from build123d import *

# Parameters (mm, degrees)
SKETCH8_R               = 35
BOSS_EXTRUDE3_DEPTH     = 1
BOSS_EXTRUDE4_START     = -53.594889
SKETCH9_R               = 5
BOSS_EXTRUDE4_DEPTH     = 113.594889
CUT_EXTRUDE2_START      = -20.791267
SKETCH10_R              = 4
CUT_EXTRUDE2_DEPTH      = 20.791267
SKETCH11_R              = 1.5
CUT_EXTRUDE3_DEPTH      = 73.971936727
BOSS_EXTRUDE5_REACH     = 74.567
SKETCH13_W              = 88.883012554
SKETCH13_H              = 5.53578549
CUT_EXTRUDE4_DEPTH      = 110.338922716
SKETCH14_R              = 1
CUT_EXTRUDE5_DEPTH      = 71.019198384
SKETCH15_W              = 75.166178786
SKETCH15_H              = 0.46421451
SKETCH15_W_2            = 75.463979311
CUT_EXTRUDE6_DEPTH      = 109.72955086
CUT_EXTRUDE7_DEPTH      = 109.707210391
CUT_EXTRUDE7_DEPTH_BACK = 109.707210391
SKETCH16_W              = 74.883691919
SKETCH16_H              = 0.2
SKETCH17_W              = 45
SKETCH17_H              = 9.670623623
CUT_EXTRUDE8_DEPTH      = 25
SKETCH18_W              = 45.166247069
SKETCH18_H              = 9.6
BOSS_EXTRUDE6_DEPTH     = 7
SKETCH19_R              = 2
CUT_EXTRUDE9_DEPTH      = 8.2
SKETCH20_W              = 85
SKETCH20_H              = 13.048799846
SKETCH20_W_2            = 85.000162577
SKETCH20_H_2            = 13.925318183
CUT_EXTRUDE10_DEPTH     = 9.6
CUT_EXTRUDE11_DEPTH     = 59.913683698
SKETCH22_R              = 5
SKETCH22_R_2            = 4.8
CUT_EXTRUDE12_DEPTH     = 10.594889107


with BuildPart() as part:
    # Sketch1 → Revolve1 (revolve)
    with BuildSketch(Plane.XY):
        with BuildLine():
            Line((-32.912878475, 10), (-22.912878475, 10))
            ThreePointArc((-22.912878475, 10), (-25, 0), (-22.912878475, -10))
            Line((-22.912878475, -10), (-32.912878475, -10))
            ThreePointArc((-32.912878475, -10), (-34.398511152, 0), (-32.912878475, 10))
        make_face()
    revolve(axis=Axis((0, 0, 0), (0, 1, 0)))

    # Sketch8 → Boss-Extrude3 (add)
    with BuildSketch(Plane.XZ.offset(10)):
        with Locations(Location((0, 0, 0), (0, 0, 270))):
            Circle(SKETCH8_R)
    extrude(amount=BOSS_EXTRUDE3_DEPTH)

    # Sketch9 → Boss-Extrude4 (add)
    with BuildSketch(Plane(origin=(0, 0, 0), x_dir=(0, 0, -1), z_dir=(1, 0, 0)).offset(BOSS_EXTRUDE4_START)):
        Circle(SKETCH9_R)
    extrude(amount=BOSS_EXTRUDE4_DEPTH)

    # Sketch10 → Cut-Extrude2 (cut)
    with BuildSketch(Plane(origin=(60, 0, 0), x_dir=(0, 0, -1), z_dir=(1, 0, 0)).offset(CUT_EXTRUDE2_START)):
        Circle(SKETCH10_R)
    extrude(amount=CUT_EXTRUDE2_DEPTH, mode=Mode.SUBTRACT)

    # Sketch11 → Cut-Extrude3 (cut, through all)
    with BuildSketch(Plane(origin=(0, 0.188776478, -4.996435073), x_dir=(-1, 0, 0), z_dir=(0, 0.03775529554410709, -0.9992870146551377))):
        with Locations(Location((-55, 0, 0), (0, 0, 90))):
            Circle(SKETCH11_R)
    extrude(amount=-CUT_EXTRUDE3_DEPTH, mode=Mode.SUBTRACT)

    # Boss-Extrude5: up to this face of the body (flat: up to its plane)
    boss_extrude5_end = Plane(part.part.faces().sort_by_distance((31.981961692, 10, 0))[0])
    # Sketch12 → Boss-Extrude5 (add, up to the picked face)
    with BuildSketch(Plane.XZ.offset(11), mode=Mode.PRIVATE) as boss_extrude5_sk1:
        Polygon((-43, -22.5), (-43, 22.5), (-16.841508162, 22.5), (-16.841508162, 28.986561578), (16.841508162, 28.986561578), (16.841508162, 22.5), (35, 22.5), (35, -22.5), (16.384759584, -22.5), (16.384759584, -28.901286862), (-16.384759584, -28.901286862), (-16.384759584, -22.5), align=None)
    boss_extrude5_tool1 = split(extrude(boss_extrude5_sk1.sketch, amount=-BOSS_EXTRUDE5_REACH, mode=Mode.PRIVATE), bisect_by=boss_extrude5_end, keep=Keep.BOTH, mode=Mode.PRIVATE)
    add(boss_extrude5_tool1.solids().sort_by(Axis((-3.565032, -11, 0.05927), (0, 1, 0)))[0])

    # Sketch13 → Cut-Extrude4 (cut, through all)
    with BuildSketch(Plane.ZY.offset(43)):
        with Locations((0, -8.232107255)):
            Rectangle(SKETCH13_W, SKETCH13_H)
        with Locations((0, 8.232107255)):
            Rectangle(SKETCH13_W, SKETCH13_H)
    extrude(amount=-CUT_EXTRUDE4_DEPTH, mode=Mode.SUBTRACT)

    # Sketch14 → Cut-Extrude5 (cut, through all)
    with BuildSketch(Plane.XZ.offset(5.46421451)):
        with Locations(Location((-32.903541804, 15.993560443, 0), (0, 0, 270))):
            Circle(SKETCH14_R)
        with Locations(Location((-32.779476251, -15.854024353, 0), (0, 0, 270))):
            Circle(SKETCH14_R)
        with Locations(Location((27.068192394, 16.122002754, 0), (0, 0, 270))):
            Circle(SKETCH14_R)
        with Locations(Location((27.449995703, -16.044926007, 0), (0, 0, 270))):
            Circle(SKETCH14_R)
    extrude(amount=-CUT_EXTRUDE5_DEPTH, mode=Mode.SUBTRACT)

    # Sketch15 → Cut-Extrude6 (cut, through all)
    with BuildSketch(Plane.ZY.offset(43)):
        with Locations((-0.380582347, 5.232107255)):
            Rectangle(SKETCH15_W, SKETCH15_H)
        with Locations((0.06827951, -5.232107255)):
            Rectangle(SKETCH15_W_2, SKETCH15_H)
    extrude(amount=-CUT_EXTRUDE6_DEPTH, mode=Mode.SUBTRACT)

    # Sketch16 → Cut-Extrude7 (cut, two sides: drawn at the far end of the back side and taken through both)
    with BuildSketch(Plane.ZY.offset(43).offset(-CUT_EXTRUDE7_DEPTH_BACK)):
        with Locations((-0.578270867, 4.9)):
            Rectangle(SKETCH16_W, SKETCH16_H)
        with Locations((-0.578270867, -4.9)):
            Rectangle(SKETCH16_W, SKETCH16_H)
    extrude(amount=CUT_EXTRUDE7_DEPTH + CUT_EXTRUDE7_DEPTH_BACK, mode=Mode.SUBTRACT)

    # Sketch17 → Cut-Extrude8 (cut)
    with BuildSketch(Plane(origin=(35, 0, 0), x_dir=(0, 0, -1), z_dir=(1, 0, 0))):
        with Locations((0, 0.035311811)):
            Rectangle(SKETCH17_W, SKETCH17_H)
    extrude(amount=CUT_EXTRUDE8_DEPTH, mode=Mode.SUBTRACT)

    # Sketch18 → Boss-Extrude6 (add)
    with BuildSketch(Plane(origin=(35, 0, 0), x_dir=(0, 0, -1), z_dir=(1, 0, 0))):
        with Locations((-0.083123535, 0)):
            Rectangle(SKETCH18_W, SKETCH18_H)
    extrude(amount=BOSS_EXTRUDE6_DEPTH)

    # Sketch19 → Cut-Extrude9 (cut)
    with BuildSketch(Plane(origin=(42, 0, 0), x_dir=(0, 0, -1), z_dir=(1, 0, 0))):
        with Locations((-16, 0.011242039)):
            Circle(SKETCH19_R)
        with Locations((16, 0.011242039)):
            Circle(SKETCH19_R)
    extrude(amount=-CUT_EXTRUDE9_DEPTH, mode=Mode.SUBTRACT)

    # Sketch20 → Cut-Extrude10 (cut)
    with BuildSketch(Plane(origin=(0, 4.8, 0), x_dir=(1, 0, 0), z_dir=(0, 1, 0))):
        with Locations((-0.5, 29.024399923)):
            Rectangle(SKETCH20_W, SKETCH20_H)
        with Locations((-0.499918711, -29.462659092)):
            Rectangle(SKETCH20_W_2, SKETCH20_H_2)
    extrude(amount=-CUT_EXTRUDE10_DEPTH, mode=Mode.SUBTRACT)

    # Sketch21 → Cut-Extrude11 (cut, through all)
    with BuildSketch(Plane.XZ.offset(4.8)):
        Polygon((-34, -8.937993072), (-34, 8.937993072), (-27.4832705, 8.937993072), (-27.4832705, 17.5), (20.384920046, 17.5), (20.384920046, 8.937993072), (33, 8.937993072), (33, -8.937993072), (20.384920046, -8.937993072), (20.384920046, -17.5), (-27.4832705, -17.5), (-27.4832705, -8.937993072), align=None)
    extrude(amount=-CUT_EXTRUDE11_DEPTH, mode=Mode.SUBTRACT)

    # Sketch22 → Cut-Extrude12 (cut)
    with BuildSketch(Plane.ZY.offset(53.594889107)):
        Circle(SKETCH22_R)
        with Locations(Location((0, 0, 0), (0, 0, 270))):
            Circle(SKETCH22_R_2, mode=Mode.SUBTRACT)
    extrude(amount=-CUT_EXTRUDE12_DEPTH, mode=Mode.SUBTRACT)


solid = part.part
Here's how the part is built. I have some questions about the finished solid (model axes, mm). A direction names the side the tool comes from. Round coordinates to 2 decimals unless told otherwise and drop trailing zeros. Write each loop counter-clockwise with the first axis right and the second up, starting at its lowest first coordinate (ties: lowest second). Pieces come first, ordered by that corner, then holes.
1. For faces 5 (the flat face through (-3, 0, -17.5)), 6 (the cylindrical face through (38, 0, 18)), 7 (the cylindrical face through (-48.37, -2.58, 4.05)), 8 (the flat face through (-1, -4.8, -20)), which set-ups out of +Z, -Z, +X, -X, +Y, -Y let a thin tool reach every point of the face, with its end or its side?
2. Suppose I cut it at C-C (z = 16). List the corners of the cut face in (x, y) for me, and give its area (3 significant figures).
3. If we mould it in two halves opening along Z, with no side actions, what happens to faces 1 (the flat face through (-1, 0, 22.5)), 2 (the flat face through (0, 0, -22.5)), 3 (the flat face through (-4, 0, 17.5)), 4 (the flat face through (-53.595, 0, 0))? For each: released by +Z, released by -Z, zero draft, split by the parting line, or undercut.
4. Will these pins go through, and if not, where does the flat tip stop? pin 1 Ø12 at (x, z) = (-23.5, -3.5) entering from +Y; pin 2 Ø5 at (y, z) = (1, 14) entering from -X; pin 3 Ø1.2 at (y, z) = (-1, 16.5) entering from +X.
5. Suppose I cut it at A-A (z = -10.5). List the corners of the cut face in (x, y) for me, and give its area (3 significant figures).
6. Suppose I cut it at D-D (z = 1). List the corners of the cut face in (x, y) for me.
7. I need wall thicknesses on L1, parallel to X at y = -3.5, z = 13; L2, parallel to Z at x = -27, y = -0.25; L3, parallel to X at y = -2.25, z = -7. Which ranges of each line are inside material? Lowest first, please.
8. Suppose I cut it at B-B (x = -16.5). List the corners of the cut face in (y, z) for me, and give its area (3 significant figures).
Answer sheet:
1. face 5: +Y, -Y
1. face 6: +X
1. face 7: -X
1. face 8: +Z, -Z, +X, -X, -Y
2. outline: (-43, -4.8) - (-33.9, -4.8) - (-33.9, 4.8) - (-43, 4.8) - close; (-31.9, -4.8) - (-27.48, -4.8) - (-27.48, 4.8) - (-31.9, 4.8) - close; (20.38, -4.8) - (26.08, -4.8) - (26.08, 4.8) - (20.38, 4.8) - close; (28.06, -4.8) - (42, -4.8) - (42, -1.99) - (33.8, -1.99) - (33.8, 2.01) - (42, 2.01) - (42, 4.8) - (28.06, 4.8) - close
2. area: 285 mm2
3. face 1: released by +Z
3. face 2: released by -Z
3. face 3: undercut
3. face 4: zero draft
4. pin 1: passes through
4. pin 2: stops at x = -43
4. pin 3: stops at x = 33.8
5. outline: (-43, -4.8) - (-27.48, -4.8) - (-27.48, 4.8) - (-43, 4.8) - close; (20.38, -4.8) - (42, -4.8) - (42, 4.8) - (20.38, 4.8) - close
5. area: 356 mm2
6. outline: (-53.59, -4.69) - (-43, -4.69) - (-43, -4.8) - (-34, -4.8) - (-34, 4.8) - (-43, 4.8) - (-43, 4.69) - (-53.59, 4.69) - close; (33, -4.8) - (42, -4.8) - (42, 4.8) - (33, 4.8) - close
7. L1: x = -43 to -27.48, 20.38 to 42
7. L2: z = -22.5 to -17.5, 17.5 to 22.5
7. L3: x = -43 to -34, 33 to 42
8. outline: (-4.8, -22.5) - (4.8, -22.5) - (4.8, -17.5) - (-4.8, -17.5) - close; (-4.8, 17.5) - (4.8, 17.5) - (4.8, 22.5) - (-4.8, 22.5) - close
8. area: 96.0 mm2
